Part model, mm, in its own coordinate system. A direction names the side the tool comes from. Give positions to 0.01 mm unless a question says otherwise; leave off trailing zeros. Loops run counter-clockwise (first coordinate to the right, second up) from the corner with the lowest first, then second, coordinate; pieces in that order, holes last. Notation, with made-up numbers: M -5.5,78 L 53.5,78 A10 ccw 53.5,87 Z; hole C 75.25,-40 d3. An arc over 180 degrees is marked long. Answer in a Markdown table with one row per item.
from build123d import *

# Parameters (mm, degrees)
PAD_DEPTH       = 14
SKETCH001_W     = 12
SKETCH001_H     = 7
PAD001_DEPTH    = 10
FILLET_R        = 4
FILLET001_R     = 6
SKETCH002_R     = 2.25
POCKET_DEPTH    = 7
SKETCH003_R     = 2.25
POCKET001_DEPTH = 41
FILLET002_R     = 4
CHAMFER_SIZE    = 1
SKETCH004_R     = 3.75
POCKET002_DEPTH = 3
SKETCH005_R     = 3.75
POCKET003_DEPTH = 3


with BuildPart() as part:
    # Sketch → Pad (new body)
    with BuildSketch(Plane.XY):
        Polygon((-20, 47), (-13, 47), (-13, 7), (13, 7), (13, 47), (20, 47), (20, 0), (-20, 0), align=None)
    extrude(amount=PAD_DEPTH)

    # Sketch001 (on Face10 of Pad) → Pad001 (join)
    with BuildSketch(Plane.XY.offset(14)):
        with Locations((0, 3.5)):
            Rectangle(SKETCH001_W, SKETCH001_H)
    extrude(amount=PAD001_DEPTH)

    # Fillet
    fillet_edges = [part.edges().sort_by_distance(p)[0] for p in [
        (-6, 3.5, 14),
        (-6, 3.5, 24),
        (6, 3.5, 24),
        (6, 3.5, 14),
    ]]
    fillet(fillet_edges, radius=FILLET_R)

    # Fillet001
    fillet001_edges = [part.edges().sort_by_distance(p)[0] for p in [
        (20, 0, 7),
        (-20, 0, 7),
        (-13, 7, 7),
        (13, 7, 7),
    ]]
    fillet(fillet001_edges, radius=FILLET001_R)

    # Sketch002 (on Face4 of Fillet001) → Pocket (cut)
    with BuildSketch(Plane.XZ):
        with Locations((0, 19)):
            Circle(SKETCH002_R)
    extrude(amount=-POCKET_DEPTH, mode=Mode.SUBTRACT)

    # Sketch003 (on Face8 of Pocket) → Pocket001 (cut)
    with BuildSketch(Plane(origin=(-20, 0, 0), x_dir=(0, -1, 0), z_dir=(-1, 0, 0))):
        with Locations((-40, 7)):
            Circle(SKETCH003_R)
    extrude(amount=-POCKET001_DEPTH, mode=Mode.SUBTRACT)

    # Fillet002
    fillet002_edges = [part.edges().sort_by_distance(p)[0] for p in [
        (16.5, 47, 14),
        (-16.5, 47, 14),
    ]]
    fillet(fillet002_edges, radius=FILLET002_R)

    # Chamfer
    chamfer_edges = [part.edges().sort_by_distance(p)[0] for p in [
        (-13, 47, 5),
        (13, 47, 5),
    ]]
    chamfer(chamfer_edges, length=CHAMFER_SIZE)

    # Sketch004 (on Face4 of Chamfer) → Pocket002 (cut)
    with BuildSketch(Plane(origin=(-20, 0, 0), x_dir=(0, -1, 0), z_dir=(-1, 0, 0))):
        with Locations((-40, 7)):
            Circle(SKETCH004_R)
    extrude(amount=-POCKET002_DEPTH, mode=Mode.SUBTRACT)

    # Sketch005 (on Face33 of Pocket002) → Pocket003 (cut)
    with BuildSketch(Plane.YZ.offset(20)):
        with Locations((40, 7)):
            Circle(SKETCH005_R)
    extrude(amount=-POCKET003_DEPTH, mode=Mode.SUBTRACT)


solid = part.part
(1) Saw through at C-C (x = 0). Write the cut outline in (y, z), plus the area to 3 significant figures.
Recorded:
| item | result |
|---|---|
| outline | M 0,0 L 7,0 L 7,16.75 L 0,16.75 Z; M 0,21.25 L 7,21.25 L 7,23 L 6,24 L 0,24 Z |
| area | 136 mm^2 |
(2) Pull direction X, two halves, no side cores. Call faces 1 (the face through (18.196, 1.711, 7.098)), 2 (the face through (14, 24, 0)), 3 (the face through (0, 7, 11)): +X half, -X half, draft (parallel to the pull), parting line (faces both ways), or undercut.
Recorded:
| item | result |
|---|---|
| face 1 | +X half |
| face 2 | draft |
| face 3 | undercut |
(3) Drill centre lines: line 1 along Z through (x, y) = (-15.85, 40); line 2 along X through (y, z) = (31.5, 11.5); line 3 along Z through (x, y) = (0, 5.5). Where is each one in solid material? Low to high.
Recorded:
| item | result |
|---|---|
| line 1 | z = 0 to 4.75, 9.25 to 14 |
| line 2 | x = -20 to -13, 13 to 20 |
| line 3 | z = 0 to 16.75, 21.25 to 24 |
(4) Pin check, flat tips, straight feed: pin 1 Ø4 at (x, z) = (-9.5, 14) entering from +Y; pin 2 Ø5 at (y, z) = (40, 7) entering from -X; pin 3 Ø11 at (x, y) = (-15, 19.5) entering from +Z. Stop position of each tip, or through.
Recorded:
| item | result |
|---|---|
| pin 1 | stops at y = 8.75 |
| pin 2 | stops at x = -17 |
| pin 3 | stops at z = 14 |
(5) Which spindle directions (+Z, -Z, +X, -X, +Y, -Y) get a long thin tool onto all of the face, cutting with end or side? Do faces 4 (the face through (-11.196, 8.711, 7.098)), 5 (the face through (12.28, 9.6, 13.28)), 6 (the face through (5.5, 6.5, 19)), 7 (the face through (17, 42, 5)). Say none if no direction does.
Recorded:
| item | result |
|---|---|
| face 4 | +Z, -Z, +Y |
| face 5 | +Z, +Y |
| face 6 | +Z, +X, +Y |
| face 7 | +X |
(6) Saw through at D-D (y = 40). Write the cut outline in (x, z), plus the area to 3 significant figures.
Recorded:
| item | result |
|---|---|
| outline | M -20,0 L -13,0 L -13,4.75 L -17,4.75 L -17,3.25 L -20,3.25 Z; M -20,10.75 L -17,10.75 L -17,9.25 L -13,9.25 L -13,13 L -14,14 L -20,14 Z; M 13,0 L 20,0 L 20,3.25 L 17,3.25 L 17,4.75 L 13,4.75 Z; M 13,9.25 L 17,9.25 L 17,10.75 L 20,10.75 L 20,14 L 14,14 L 13,13 Z |
| area | 114 mm^2 |
(7) Saw through at A-A (y = 15.5). Write the cut outline in (x, z).
Recorded:
| item | result |
|---|---|
| outline | M -20,0 L -13,0 L -13,13 L -14,14 L -20,14 Z; M 13,0 L 20,0 L 20,14 L 14,14 L 13,13 Z |
(8) Saw through at B-B (z = 7). Give the number of separate pieces and of enclosed holes in the cut face, plus the area to 3 significant figures.
Recorded:
| item | result |
|---|---|
| separate pieces | 3 |
| enclosed holes | 0 |
| area | 758 mm^2 |
